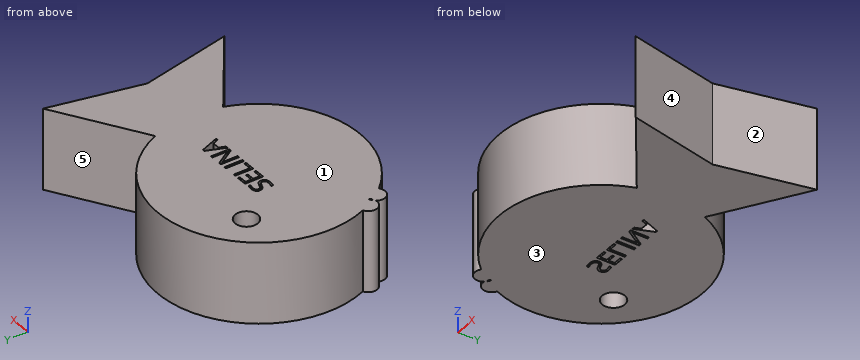
from build123d import *

# Parameters (mm, degrees)
F0_R     = 1.4016050998
F0_W     = 0.2615615931
F0_H     = 2.2506119
F1_DEPTH = 10


with BuildPart() as f1:
    # F0 (on Top) → F1 (new body)
    with BuildSketch(Plane.XY):
        with BuildLine():
            ThreePointArc((15.6497281832, -3.8894937424), (16.1141499311, -1.9693410977), (16.2702568807, 0))
            ThreePointArc((16.2702568807, 0), (16.0296169984, 2.440919807), (15.31696256, 4.7878583893))
            ThreePointArc((15.31696256, 4.7878583893), (-1.0286524493, 11.5421171906), (-7.7672612448, -4.8099558734))
            ThreePointArc((-7.7672612448, -4.8099558734), (-6.7093134723, -4.877150661), (-6.1988012008, -5.8062070906))
            ThreePointArc((-6.1988012008, -5.8062070906), (-6.2518108787, -6.1436650731), (-6.4057336913, -6.4486170097))
            ThreePointArc((-6.4057336913, -6.4486170097), (-5.4828783131, -6.684585858), (-5.0770177625, -7.5463402081))
            ThreePointArc((-5.0770177625, -7.5463402081), (-5.1829933682, -8.0214071787), (-5.4808256952, -8.4063946597))
            ThreePointArc((-5.4808256952, -8.4063946597), (6.3832446914, -12.2238412417), (15.6497281832, -3.8894937424))
        make_face()
        with Locations((-2.2391737439, 5.7797180489)):
            Circle(F0_R, mode=Mode.SUBTRACT)
        with BuildLine():
            add(Edge.make_bspline(
                [(2.4462237992, 0.9743292489), (2.5792212194, 0.8295098358), (2.5792212194, 0.598980974)],
                knots=[0, 0, 0, 1, 1, 1], degree=2))
            add(Edge.make_bspline(
                [(2.5792212194, 0.598980974), (2.5792212194, 0.3019534022), (2.3637161403, 0.1354603354)],
                knots=[0, 0, 0, 1, 1, 1], degree=2))
            add(Edge.make_bspline(
                [(2.3637161403, 0.1354603354), (2.1482110613, -0.0310327314), (1.7787737829, -0.0310327314)],
                knots=[0, 0, 0, 1, 1, 1], degree=2))
            add(Edge.make_bspline(
                [(1.7787737829, -0.0310327314), (1.3787963561, -0.0310327314), (1.1630449855, 0.0724097066)],
                knots=[0, 0, 0, 1, 1, 1], degree=2))
            Line((1.1630449855, 0.0724097066), (1.1630449855, 0.324612222))
            add(Edge.make_bspline(
                [(1.1630449855, 0.324612222), (1.3019534022, 0.2664874235), (1.4649983877, 0.2324991939)],
                knots=[0, 0, 0, 1, 1, 1], degree=2))
            add(Edge.make_bspline(
                [(1.4649983877, 0.2324991939), (1.6280433733, 0.1985109643), (1.7881328606, 0.1985109643)],
                knots=[0, 0, 0, 1, 1, 1], degree=2))
            add(Edge.make_bspline(
                [(1.7881328606, 0.1985109643), (2.0496944537, 0.1985109643), (2.1821992909, 0.2977664464)],
                knots=[0, 0, 0, 1, 1, 1], degree=2))
            add(Edge.make_bspline(
                [(2.1821992909, 0.2977664464), (2.3147041281, 0.3970219285), (2.3147041281, 0.5743518222)],
                knots=[0, 0, 0, 1, 1, 1], degree=2))
            add(Edge.make_bspline(
                [(2.3147041281, 0.5743518222), (2.3147041281, 0.6910940021), (2.2676624479, 0.7657203324)],
                knots=[0, 0, 0, 1, 1, 1], degree=2))
            add(Edge.make_bspline(
                [(2.2676624479, 0.7657203324), (2.2206207678, 0.8403466626), (2.1105284589, 0.903643583)],
                knots=[0, 0, 0, 1, 1, 1], degree=2))
            add(Edge.make_bspline(
                [(2.1105284589, 0.903643583), (2.0004361499, 0.9669405033), (1.7758182846, 1.0467389555)],
                knots=[0, 0, 0, 1, 1, 1], degree=2))
            add(Edge.make_bspline(
                [(1.7758182846, 1.0467389555), (1.4620428895, 1.1590478881), (1.3273214287, 1.3129800874)],
                knots=[0, 0, 0, 1, 1, 1], degree=2))
            add(Edge.make_bspline(
                [(1.3273214287, 1.3129800874), (1.1925999678, 1.4669122868), (1.1925999678, 1.7146815548)],
                knots=[0, 0, 0, 1, 1, 1], degree=2))
            add(Edge.make_bspline(
                [(1.1925999678, 1.7146815548), (1.1925999678, 1.9747653988), (1.3879091423, 2.1286975981)],
                knots=[0, 0, 0, 1, 1, 1], degree=2))
            add(Edge.make_bspline(
                [(1.3879091423, 2.1286975981), (1.5832183168, 2.2826297975), (1.9053676236, 2.2826297975)],
                knots=[0, 0, 0, 1, 1, 1], degree=2))
            add(Edge.make_bspline(
                [(1.9053676236, 2.2826297975), (2.2408166724, 2.2826297975), (2.52257417, 2.159484038)],
                knots=[0, 0, 0, 1, 1, 1], degree=2))
            Line((2.52257417, 2.159484038), (2.4408053858, 1.9319106745))
            add(Edge.make_bspline(
                [(2.4408053858, 1.9319106745), (2.1620033863, 2.0486528545), (1.8989640441, 2.0486528545)],
                knots=[0, 0, 0, 1, 1, 1], degree=2))
            add(Edge.make_bspline(
                [(1.8989640441, 2.0486528545), (1.6910940021, 2.0486528545), (1.5741055306, 1.9594953246)],
                knots=[0, 0, 0, 1, 1, 1], degree=2))
            add(Edge.make_bspline(
                [(1.5741055306, 1.9594953246), (1.4571170591, 1.8703377948), (1.4571170591, 1.7117260566)],
                knots=[0, 0, 0, 1, 1, 1], degree=2))
            add(Edge.make_bspline(
                [(1.4571170591, 1.7117260566), (1.4571170591, 1.5949838766), (1.500218075, 1.5201112549)],
                knots=[0, 0, 0, 1, 1, 1], degree=2))
            add(Edge.make_bspline(
                [(1.500218075, 1.5201112549), (1.5433190908, 1.4452386331), (1.6457763626, 1.3829268788)],
                knots=[0, 0, 0, 1, 1, 1], degree=2))
            add(Edge.make_bspline(
                [(1.6457763626, 1.3829268788), (1.7482336345, 1.3206151245), (1.9590591747, 1.2452499197)],
                knots=[0, 0, 0, 1, 1, 1], degree=2))
            add(Edge.make_bspline(
                [(1.9590591747, 1.2452499197), (2.3132263789, 1.119148662), (2.4462237992, 0.9743292489)],
                knots=[0, 0, 0, 1, 1, 1], degree=2))
        make_face(mode=Mode.SUBTRACT)
        Polygon((4.2943953572, 0.233976943), (4.2943953572, 0), (3.0397863598, 0), (3.0397863598, 2.2506119), (4.2943953572, 2.2506119), (4.2943953572, 2.0181127061), (3.3013479529, 2.0181127061), (3.3013479529, 1.2930304744), (4.2343002266, 1.2930304744), (4.2343002266, 1.0620090296), (3.3013479529, 1.0620090296), (3.3013479529, 0.233976943), align=None, mode=Mode.SUBTRACT)
        Polygon((6.047498389, 0), (4.7928893916, 0), (4.7928893916, 2.2506119), (5.0544509847, 2.2506119), (5.0544509847, 0.2369324412), (6.047498389, 0.2369324412), align=None, mode=Mode.SUBTRACT)
        with Locations((6.5600310399, 1.12530595)):
            Rectangle(F0_W, F0_H, mode=Mode.SUBTRACT)
        with BuildLine():
            Line((9.066047245, 2.2506119), (9.066047245, 0))
            Line((9.066047245, 0), (8.7675419241, 0))
            Line((8.7675419241, 0), (7.5375620785, 1.8885633672))
            Line((7.5375620785, 1.8885633672), (7.5252475026, 1.8885633672))
            add(Edge.make_bspline(
                [(7.5252475026, 1.8885633672), (7.5498766545, 1.5560698166), (7.5498766545, 1.2792381493)],
                knots=[0, 0, 0, 1, 1, 1], degree=2))
            Line((7.5498766545, 1.2792381493), (7.5498766545, 0))
            Line((7.5498766545, 0), (7.3080183829, 0))
            Line((7.3080183829, 0), (7.3080183829, 2.2506119))
            Line((7.3080183829, 2.2506119), (7.6035682056, 2.2506119))
            Line((7.6035682056, 2.2506119), (8.8305925529, 0.3694372784))
            Line((8.8305925529, 0.3694372784), (8.8429071289, 0.3694372784))
            add(Edge.make_bspline(
                [(8.8429071289, 0.3694372784), (8.8399516307, 0.4108142536), (8.8291148038, 0.6364172849)],
                knots=[0, 0, 0, 1, 1, 1], degree=2))
            add(Edge.make_bspline(
                [(8.8291148038, 0.6364172849), (8.818277977, 0.8620203163), (8.8212334752, 0.9590591747)],
                knots=[0, 0, 0, 1, 1, 1], degree=2))
            Line((8.8212334752, 0.9590591747), (8.8212334752, 2.2506119))
            Line((8.8212334752, 2.2506119), (9.066047245, 2.2506119))
        make_face(mode=Mode.SUBTRACT)
        Polygon((11.3703506962, 0), (11.0994300253, 0), (10.8191502768, 0.715723154), (9.9172307345, 0.715723154), (9.6403990672, 0), (9.3753893928, 0), (10.2649943592, 2.2599709777), (10.4851789771, 2.2599709777), align=None, mode=Mode.SUBTRACT)
        with BuildLine():
            ThreePointArc((15.31696256, 4.7878583893), (16.0296169984, 2.440919807), (16.2702568807, 0))
            ThreePointArc((16.2702568807, 0), (16.1141499311, -1.9693410977), (15.6497281832, -3.8894937424))
            Line((15.6497281832, -3.8894937424), (25.9802397341, -11.2746227533))
            Line((25.9802397341, -11.2746227533), (23.5263779759, 0))
            Line((23.5263779759, 0), (25.9188935161, 11.3009084016))
            Line((25.9188935161, 11.3009084016), (15.31696256, 4.7878583893))
        make_face()
        with BuildLine():
            ThreePointArc((-6.1988012008, -5.8062070906), (-6.7093134723, -4.877150661), (-7.7672612448, -4.8099558734))
            ThreePointArc((-7.7672612448, -4.8099558734), (-7.3353744108, -5.7371555337), (-6.8291260147, -6.6259401022))
            ThreePointArc((-6.8291260147, -6.6259401022), (-6.6266300861, -6.5153112644), (-6.4057336913, -6.4486170097))
            ThreePointArc((-6.4057336913, -6.4486170097), (-6.2518108787, -6.1436650731), (-6.1988012008, -5.8062070906))
        make_face()
        with BuildLine():
            ThreePointArc((-6.8291260147, -6.6259401022), (-7.3353744108, -5.7371555337), (-7.7672612448, -4.8099558734))
            ThreePointArc((-7.7672612448, -4.8099558734), (-8.3471428725, -6.1433715274), (-7.0984216701, -6.8883247926))
            ThreePointArc((-7.0984216701, -6.8883247926), (-6.9748850194, -6.7457286125), (-6.8291260147, -6.6259401022))
        make_face()
        with BuildLine():
            ThreePointArc((-7.0984216701, -6.8883247926), (-6.9597521838, -8.3614224908), (-5.4808256952, -8.4063946597))
            ThreePointArc((-5.4808256952, -8.4063946597), (-6.1476298332, -7.608253619), (-6.7457763686, -6.7574436512))
            ThreePointArc((-6.7457763686, -6.7574436512), (-6.9164663705, -6.8380607946), (-7.0984216701, -6.8883247926))
        make_face()
        with BuildLine():
            ThreePointArc((-6.7457763686, -6.7574436512), (-6.1476298332, -7.608253619), (-5.4808256952, -8.4063946597))
            ThreePointArc((-5.4808256952, -8.4063946597), (-5.1829933682, -8.0214071787), (-5.0770177625, -7.5463402081))
            ThreePointArc((-5.0770177625, -7.5463402081), (-5.4828783131, -6.684585858), (-6.4057336913, -6.4486170097))
            ThreePointArc((-6.4057336913, -6.4486170097), (-6.5594644952, -6.6209675039), (-6.7457763686, -6.7574436512))
        make_face()
        with BuildLine():
            ThreePointArc((-6.7457763686, -6.7574436512), (-6.7876559356, -6.6918216476), (-6.8291260147, -6.6259401022))
            ThreePointArc((-6.8291260147, -6.6259401022), (-6.9748850194, -6.7457286125), (-7.0984216701, -6.8883247926))
            ThreePointArc((-7.0984216701, -6.8883247926), (-6.9164663705, -6.8380607946), (-6.7457763686, -6.7574436512))
        make_face()
    extrude(amount=F1_DEPTH)


solid = f1.part
Input: part model. Units: mm. Frame: model coordinates. Face numbers are marked on the shaded views. A direction names the side the tool comes from. Coordinates: 2 decimals unless noted, no trailing zeros. Loops run counter-clockwise (first coordinate to the right, second up) from the corner with the lowest first, then second, coordinate; pieces in that order, holes last. Notation, with made-up numbers: (77.25, 40.25) - (107.25, 40.25) arc R3 cw to (107.25, 44.25) - close; hole circle Ø9 at (-36, -8.75). An arc over 180 degrees is marked (long way). Answer in a Markdown table with one row per item. Add a question column.
Item 1: Section query B-B on y = -7.75. Return the cut outline in (x, z).
Item 2: Mould query, pull axis X, two halves, no side actions, for the marked faces 3, 4 and 5. Classes: released by +X, released by -X, zero draft, split by the parting line, or undercut.
Item 3: Section query A-A on y = 7.75. Return the cut outline in (x, z).
Item 4: Contact query for flat-ended pins moving along their axis: P1, Ø1.8, axis at y = 1.5, z = 7, coming from the +X side; P2, Ø2, axis at y = -10, z = 4.5, coming from the -X side; P3, Ø6, axis at x = 19, z = 2, coming from the -Y side; P4, Ø3, axis at x = 18, y = 9.5, coming from the +Z side. Output: stop coordinate, or through.
Item 5: Section query C-C on x = 13. Return the cut outline in (y, z).
Item 6: Line query: line 1 along X through (y, z) = (6.5, 2); line 2 along Y through (x, z) = (-2, 3); line 3 along X through (y, z) = (9, 6.5). Output: solid intervals per line, ascending. Write a range as [from, to].
Item 7: Access query for the marked faces 1 and 2. Directions: +Z, -Z, +X, -X, +Y, -Y. A direction counts if a zero-diameter tool reaches every point of the face in a straight line with its end or side. Return the directions, or none.
Item 8: Section query D-D on z = 5. State how many separate pieces and enclosed holes the cut face has, then the cut area to 3 significant figures.
Recorded:
| question | item | result |
|---|---|---|
| 1 | outline | (-7.29, 0) - (13.58, 0) - (13.58, 10) - (-7.29, 10) - close; (21.05, 0) - (25.21, 0) - (25.21, 10) - (21.05, 10) - close |
| 2 | face 3 | zero draft |
| 2 | face 4 | released by +X |
| 2 | face 5 | undercut |
| 3 | outline | (-6.04, 0) - (13.58, 0) - (13.58, 10) - (-6.04, 10) - close; (20.14, 0) - (25.17, 0) - (25.17, 10) - (20.14, 10) - close |
| 4 | P1 | x = 24.03 |
| 4 | P2 | x = -4.9 |
| 4 | P3 | y = -8.43 |
| 4 | P4 | through |
| 5 | outline | (-8.43, 0) - (8.43, 0) - (8.43, 10) - (-8.43, 10) - close |
| 6 | line 1 | [-6.91, -3.44], [-1.04, 14.45], [18.1, 24.9] |
| 6 | line 2 | [-11.09, 4.4], [7.16, 11.09] |
| 6 | line 3 | [-4.9, 12.44], [22.17, 25.43] |
| 7 | face 1 | +Z, +X, -X, +Y, -Y |
| 7 | face 2 | +Z, -Z, +X |
| 8 | separate pieces | 1 |
| 8 | enclosed holes | 8 |
| 8 | area | 613 mm^2 |
